Geometry: see drawing. Coordinates: mm, zero at the bounding-box minimum. A direction names the side the tool comes from. Round coordinates to 2 decimals unless told otherwise and drop trailing zeros. Order: outer loops, then holes, each group sorted by start corner. A loop starts at its lowest first (then second) coordinate and runs counter-clockwise, first axis right, second up. Notation, with made-up numbers: (18, -26.75) -> (58, -26.75) arc R13 cw to (58, -1.75) -> close; hole circle Ø3 at (68.5, 14.5). An arc over 180 degrees is marked (long way). Put each result on its own line as item: value.
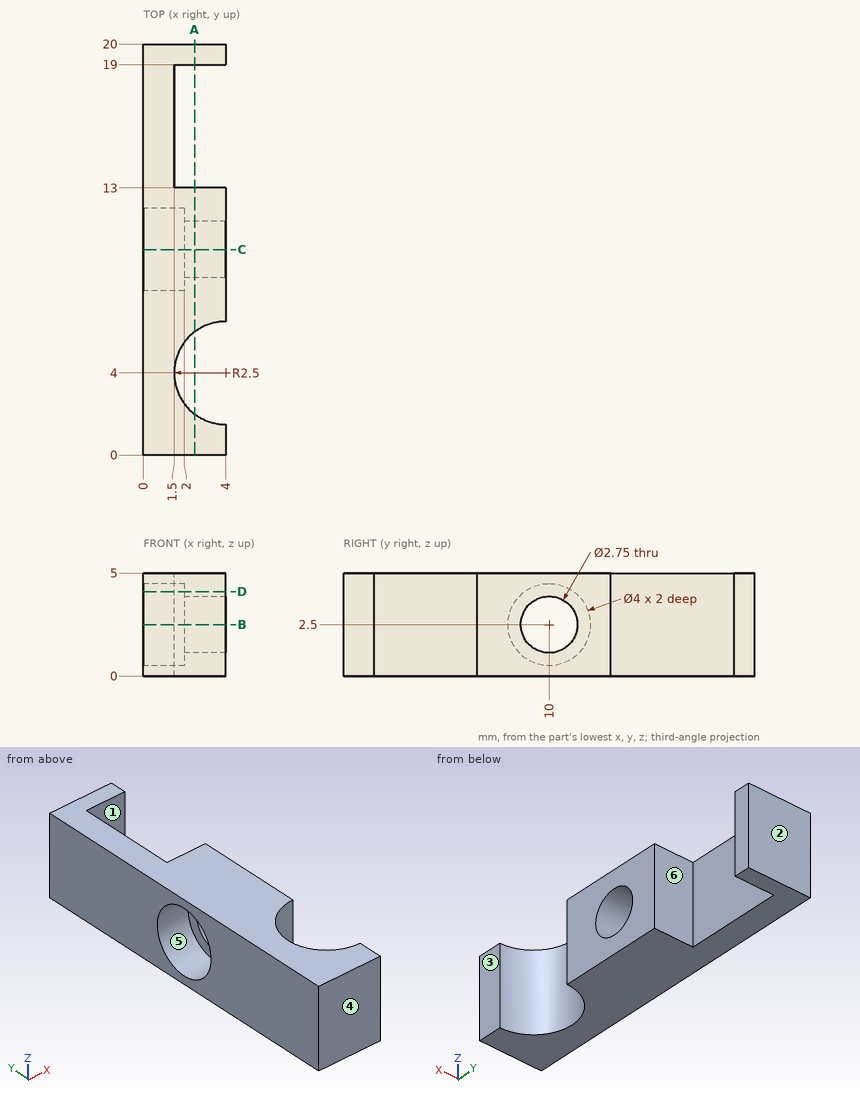
1. Set-up query: the marked faces 1 and 2. Return all of +Z, -Z, +X, -X, +Y, -Y with unobstructed straight access to the full face (end or side cutting, diameter ignored); none if empty.
Ans:
face 1: +Z, -Z, +X
face 2: +Z, -Z, +X, -X, +Y
2. Cut plane C-C on y = 10. Return loops of the section in (x, z) (3 decimals).
Ans:
outline: (0, 0) -> (4, 0) -> (4, 1.125) -> (2, 1.125) -> (2, 0.5) -> (0, 0.5) -> close; (0, 4.5) -> (2, 4.5) -> (2, 3.875) -> (4, 3.875) -> (4, 5) -> (0, 5) -> close
3. Contact query for a flat-ended pin moving along its axis: P1, Ø2.5, axis at y = 15.5, z = 1.5, coming from the +X side. Output: stop coordinate, or through.
Ans:
P1: x = 1.5
4. Cut plane B-B on z = 2.5. Return loops of the section in (x, y) (3 decimals).
Ans:
outline: (0, 0) -> (4, 0) -> (4, 1.5) arc R2.5 cw to (4, 6.5) -> (4, 8.625) -> (2, 8.625) -> (2, 8) -> (0, 8) -> close; (0, 12) -> (2, 12) -> (2, 11.375) -> (4, 11.375) -> (4, 13) -> (1.5, 13) -> (1.5, 19) -> (4, 19) -> (4, 20) -> (0, 20) -> close
5. Material intervals for probe 1 along Y at (x, z) = (2.85, 0.9); probe 2 along Y at (x, z) = (2.95, 1.8); probe 3 along Y at (x, z) = (2.1, 3.95), sorted ascending.
Ans:
probe 1: 0 to 1.78, 6.22 to 13, 19 to 20
probe 2: 0 to 1.73, 6.27 to 8.82, 11.18 to 13, 19 to 20
probe 3: 0 to 2.38, 5.62 to 13, 19 to 20
6. Cut plane D-D on z = 4.1. Return loops of the section in (x, y).
Ans:
outline: (0, 0) -> (4, 0) -> (4, 1.5) arc R2.5 cw to (4, 6.5) -> (4, 13) -> (1.5, 13) -> (1.5, 19) -> (4, 19) -> (4, 20) -> (0, 20) -> (0, 11.2) -> (2, 11.2) -> (2, 8.8) -> (0, 8.8) -> close
7. Cut plane A-A on x = 2.5. Return loops of the section in (y, z) (3 decimals).
Ans:
outline: (0, 0) -> (2, 0) -> (2, 5) -> (0, 5) -> close; (6, 0) -> (13, 0) -> (13, 5) -> (6, 5) -> close; (19, 0) -> (20, 0) -> (20, 5) -> (19, 5) -> close; hole circle Ø2.75 at (10, 2.5)
8. Draft query along Y for the marked faces 3, 4, 5 and 6. Return one class per face: +Y half, -Y half, draft (parallel to the pull), parting line (faces both ways), or undercut.
Ans:
face 3: draft
face 4: -Y half
face 5: undercut
face 6: undercut
